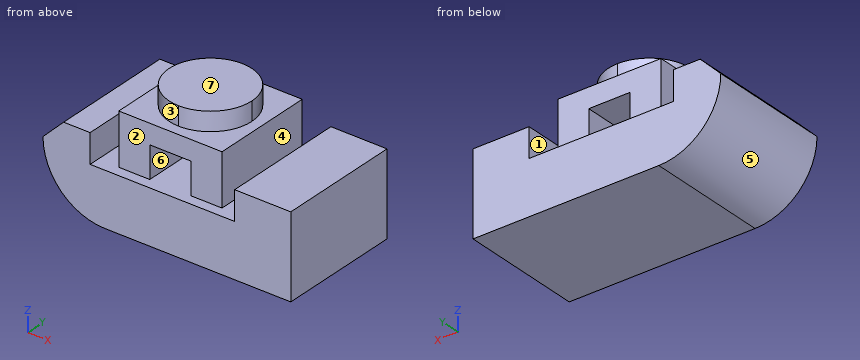
```python
from build123d import *

# Parameters (mm, degrees)
F1_DEPTH = 30
F2_DEPTH = 25
F0_W     = 40
F0_H     = 9.0879101008
F3_DEPTH = 20
F4_R     = 30
F5_SIZE  = 9.99999
F6_R     = 19.99999


# Not quite as in the source:
# - a fillet or chamfer is up to 0.001 mm smaller than in the source, because OpenCascade refuses the exact size


with BuildPart() as f1:
    # F0 (on Front) → F1 (new body, symmetric)
    with BuildSketch(Plane.XZ):
        Polygon((-57.820021317, -12.9469532817), (-35, -12.9469532817), (-35, 12.9469532817), (-35, 27.0530467183), (-57.820021317, 27.0530467183), align=None)
        Polygon((-35, -12.9469532817), (35, -12.9469532817), (35, 12.9469532817), (25, 12.9469532817), (10, 12.9469532817), (-10, 12.9469532817), (-25, 12.9469532817), (-35, 12.9469532817), align=None)
        Polygon((35, 12.9469532817), (35, -12.9469532817), (62.179978683, -12.9469532817), (62.179978683, 27.0530467183), (35, 27.0530467183), align=None)
    extrude(amount=F1_DEPTH, both=True)

    # F0 (on Front) → F2 (join, symmetric)
    with BuildSketch(Plane.XZ):
        Polygon((10, 12.9469532817), (25, 12.9469532817), (25, 37.9469532817), (20, 37.9469532817), (-20, 37.9469532817), (-25, 37.9469532817), (-25, 12.9469532817), (-10, 12.9469532817), (-10, 28.3428579569), (10, 28.3428579569), align=None)
    extrude(amount=F2_DEPTH, both=True)

    # F0 (on Front) → F3 (join, symmetric)
    with BuildSketch(Plane.XZ):
        with Locations((0, 42.4909083322)):
            Rectangle(F0_W, F0_H)
    extrude(amount=F3_DEPTH, both=True)

    # F4
    f4_edges = [f1.edges().sort_by_distance(p)[0] for p in [
        (-57.820021, 0, -12.946953),
    ]]
    fillet(f4_edges, radius=F4_R)

    # F5 (size 10 in the source; OpenCascade refuses exactly that, so slightly less here)
    f5_edges = [f1.edges().sort_by_distance(p)[0] for p in [
        (-57.820021, 0, 27.053047),
    ]]
    chamfer(f5_edges, length=F5_SIZE)

    # F6 (radius 20 in the source; OpenCascade refuses exactly that, so slightly less here)
    f6_edges = [f1.edges().sort_by_distance(p)[0] for p in [
        (20, -20, 42.490908),
        (20, 20, 42.490908),
        (-20, -20, 42.490908),
        (-20, 20, 42.490908),
    ]]
    fillet(f6_edges, radius=F6_R)


solid = f1.part
```
For this review, take the finished solid that the model builds, in its own axes (mm). Face numbers are marked on the shaded views. A direction names the side the tool comes from. Coordinates: 2 decimals unless noted, no trailing zeros. Write each loop counter-clockwise with the first axis right and the second up, starting at its lowest first coordinate (ties: lowest second). Pieces come first, ordered by that corner, then holes.
(1) Wall thickness on probe 1 along Z at (x, y) = (-4, 21); probe 2 along Z at (x, y) = (40, -18); probe 3 along Z at (x, y) = (5.5, 18.5): over which ranges is each line inside the solid? List them lowest first.
(2) For pin 1 Ø12.5 at (y, z) = (8.5, 22.5) entering from -X; pin 2 Ø2 at (y, z) = (3.5, 38) entering from +X; pin 3 Ø1 at (x, y) = (-39.5, 5.5) entering from +Z; pin 4 Ø12.5 at (x, z) = (-8, 31.5) entering from +Y, all flat-tipped, find the tip position at first contact; note any pin that passes through.
(3) Add section C-C on x = -8.5. Give the boundary of the cut face in (y, z), then the cut area to 3 significant figures.
(4) Add section D-D on z = 19. Give the boundary of the cut face in (x, y).
(5) The part is to be moulded in two halves that separate along Z. For the marked faces 4, 5, 6 and 7, say which applies: +Z half, -Z half, draft (parallel to the pull), parting line (faces both ways), or undercut.
(6) Tool access review of the marked faces 1, 2 and 3: name each direction out of +Z, -Z, +X, -X, +Y, -Y from which nothing blocks a thin tool from reaching the whole face with its end or side.
Answer sheet:
1. probe 1: z = -12.95 to 12.95, 28.34 to 37.95
1. probe 2: z = -12.95 to 27.05
1. probe 3: z = -12.95 to 12.95, 28.34 to 47.03
2. pin 1: stops at x = -57.82
2. pin 2: stops at x = 25
2. pin 3: stops at z = 27.05
2. pin 4: stops at y = 25
3. outline: (-30, -12.95) - (30, -12.95) - (30, 12.95) - (-30, 12.95) - close; (-25, 28.34) - (25, 28.34) - (25, 37.95) - (18.1, 37.95) - (18.1, 47.03) - (-18.1, 47.03) - (-18.1, 37.95) - (-25, 37.95) - close
3. area: 2,360 mm2
4. outline: (-55.87, -30) - (-35, -30) - (-35, 30) - (-55.87, 30) - close; (-25, -25) - (-10, -25) - (-10, 25) - (-25, 25) - close; (10, -25) - (25, -25) - (25, 25) - (10, 25) - close; (35, -30) - (62.18, -30) - (62.18, 30) - (35, 30) - close
5. face 4: draft
5. face 5: -Z half
5. face 6: undercut
5. face 7: +Z half
6. face 1: +Z, +Y, -Y
6. face 2: +Z, -Y
6. face 3: +Z, -X, -Y
